Autodesk Inventor part; units mm, degrees
ref_plane "YZ Plane" through (0, 0, 0) normal (1, 0, 0) x (0, 1, 0)
ref_plane "XZ Plane" through (0, 0, 0) normal (0, 1, 0) x (-1, 0, 0)
ref_plane "XY Plane" through (0, 0, 0) normal (0, 0, 1) x (1, 0, 0)
sketch "Boceto1" plane through (0, 0, 0) normal (0, 1, 0) x (-1, 0, 0)
  line L0 (0, 0) -> (50, 0)
  line L1 (50, 0) -> (50, -50)
  line L2 (50, -50) -> (0, -50)
  line L3 (0, -50) -> (0, 0)
  line L4 (1.5, -48.5) -> (48.5, -48.5)
  line L5 (48.5, -48.5) -> (48.5, -1.5)
  line L6 (48.5, -1.5) -> (1.5, -1.5)
  line L7 (1.5, -1.5) -> (1.5, -48.5)
  line L8 (1.5, -48.5) -> (48.5, -1.5) construction
  line L9 (48.5, -48.5) -> (1.5, -1.5) construction
  point P0 (25, -25)
  dimension "d0" = 50
  dimension "d1" = 50
  dimension "d6" = 1.5
  dimension "d7" = 1.5
  dimension "d8" = 1.5
  dimension "d9" = 1.5
extrude "Extrusión1" add sketch "Boceto1" along normal blind 1690.856
equation "\"d0\" = d1"
equation "\"d7\" = d6"
equation "\"d8\" = d6"
equation "\"d9\" = d6"
properties part number "Mesa_base3"
The model under review builds one solid part; all positions refer to its coordinate system, in mm. A direction names the side the tool comes from. Round coordinates to 2 decimals unless told otherwise and drop trailing zeros. Loops run counter-clockwise (first coordinate to the right, second up) from the corner with the lowest first, then second, coordinate; pieces in that order, holes last. Notation, with made-up numbers: (-16.75, 80.5) -> (35.25, 80.5) arc R27 ccw to (35.25, 106.5) -> close; hole circle Ø11 at (60, 41). An arc over 180 degrees is marked (long way). Answer as a JSON object with one key per item and string values. Group by question number.
1) Mouldability with a two-part tool opening along Z and no side actions: class faces 1 (the face through (-25, 834, -50)), 2 (the face through (-23, 1690.856, -49)), 3 (the face through (-1.5, 834, -25)) as released by +Z, released by -Z, zero draft, split by the parting line, or undercut.
2) We need section B-B on y = 541. Write out the cut boundary in (x, z), then the cut area to 3 significant figures.
3) We need section A-A on x = -25. Write out the cut boundary in (y, z), then the cut area to 3 significant figures.
4) We need section C-C on z = -35. Write out the cut boundary in (x, y), then the cut area to 3 significant figures.
5) For faces 4 (the face through (-25, 834, -48.5)), 5 (the face through (-25, 834, 0)), list the 3-axis set-ups (+Z, -Z, +X, -X, +Y, -Y) from which the entire face can be reached by the end or side of a thin tool; tool diameter is ignored.
6) For line 1 (Z direction, x = -2, y = 1316.5), list the stretches that pass through material, from the lowest coordinate up. Write a range as [from, to].
Result set:
{
 "1": {"face 1": "released by -Z", "face 2": "zero draft", "face 3": "undercut"},
 "2": {"outline": "(-50, -50) -> (0, -50) -> (0, 0) -> (-50, 0) -> close; hole (-48.5, -48.5) -> (-1.5, -48.5) -> (-1.5, -1.5) -> (-48.5, -1.5) -> close", "area": "291 mm²"},
 "3": {"outline": "(0, -50) -> (1690.86, -50) -> (1690.86, -48.5) -> (0, -48.5) -> close; (0, -1.5) -> (1690.86, -1.5) -> (1690.86, 0) -> (0, 0) -> close", "area": "5,070 mm²"},
 "4": {"outline": "(-50, 0) -> (-48.5, 0) -> (-48.5, 1690.86) -> (-50, 1690.86) -> close; (-1.5, 0) -> (0, 0) -> (0, 1690.86) -> (-1.5, 1690.86) -> close", "area": "5,070 mm²"},
 "5": {"face 4": "+Y, -Y", "face 5": "+Z, +X, -X, +Y, -Y"},
 "6": {"line 1": "[-50, -48.5], [-1.5, 0]"}
}
